Design review of the part built by this model. Coordinates are the model's own, in mm. A direction names the side the tool comes from. Give positions to 0.01 mm unless a question says otherwise; leave off trailing zeros. Order: outer loops, then holes, each group sorted by start corner. A loop starts at its lowest first (then second) coordinate and runs counter-clockwise, first axis right, second up. Notation, with made-up numbers: (26.25, 6.25) -> (34.25, 6.25) arc R16 ccw to (34.25, 35.25) -> close; hole circle Ø4 at (13, 5). An arc over 180 degrees is marked (long way). One line per item, written item: value. Start each with the question number.
1) Consider section B-B (z = 87.5). State the section outline as (x, y) points, plus the area to 3 significant figures.
2) The part is to be moulded in two halves that separate along X. For faces 4 (the face through (16.421, -2.535, 26.862)), 5 (the face through (11.68, -1.36, 7)), 6 (the face through (5.625, -3, 44)), say which applies: released by +X, released by -X, zero draft, split by the parting line, or undercut.
3) Tool access review of faces 1 (the face through (12.47, -2.535, 73.859)), 2 (the face through (12.47, -2.465, 86.792)), 3 (the face through (5.625, -2, 80)): name each direction out of +Z, -Z, +X, -X, +Y, -Y from which nothing blocks a thin tool from reaching the whole face with its end or side.
4) Wall thickness on line 1 along Z through (x, y) = (2.5, -3.2); line 2 along Z through (x, y) = (2, -4.25); line 3 along Z through (x, y) = (13, -1.2): over which ranges is each line inside the solid? List them lowest first. Write a range as from..to.
5) Consider section C-C (x = 15). State how many separate pieces and enclosed holes the cut face has, plus the area to 3 significant figures.
6) For pin 1 (2.5 mm diameter, centred on y = -2.5, z = 43.5, fed in from +X); pin 2 (8 mm diameter, centred on x = 14.5, z = 76.5, fed in from +Y); pin 3 (1.2 mm diameter, centred on x = 2.63, z = 11.83, fed in from +Y); pin 4 (4 mm diameter, centred on x = 12.38, z = 8.33, fed in from -Y), all flat-tipped, find the tip position at first contact; note any pin that passes through.
7) Consider section D-D (z = 65). State the section outline as (x, y) points, plus the area to 3 significant figures.
8) Consider section A-A (x = 7.25). State the section outline as (y, z) points.
from build123d import *

# Parameters (mm, degrees)
F1_DEPTH        = 5
F4_DEPTH        = 13.5
F6_DEPTH        = 7.5
F8_DEPTH        = 6.5
F10_D           = 3
F10_CSINK_D     = 7.5
F10_CSINK_ANGLE = 90
F12_D           = 2
F12_CSINK_D     = 5
F12_CSINK_ANGLE = 90


with BuildPart() as f1:
    # F0 (on Front) → F1 (new body)
    with BuildSketch(Plane.XZ):
        Polygon((19.12546, 114.327021), (-0.37454, 114.327021), (-0.37454, -0.672979), (19.62546, -0.672979), (19.62546, 29.327021), (13.12546, 29.327021), (13.12546, 39.827021), (5.62546, 39.827021), (5.62546, 48.327021), (19.12546, 48.327021), (19.12546, 75.827021), (5.62546, 75.827021), (5.62546, 84.327021), (19.12546, 84.327021), align=None)
    extrude(amount=F1_DEPTH)

    # F2 (on face) + F3 (on face) → F4 (cut)
    with BuildSketch(Plane.YZ.offset(19.12546)):
        Polygon((-5, 84.327021), (0, 84.327021), (-5, 89.327021), align=None)
    with BuildSketch(Plane.YZ.offset(19.12546)):
        Polygon((0, 75.827021), (-5, 75.827021), (0, 71.834676), align=None)
        Polygon((0, 53.327021), (-5, 48.327021), (0, 48.327021), align=None)
    extrude(amount=-F4_DEPTH, mode=Mode.SUBTRACT)

    # F5 (on face) → F6 (cut)
    with BuildSketch(Plane.YZ.offset(13.12546)):
        Polygon((-5, 34.827021), (0, 39.827021), (-5, 39.827021), align=None)
    extrude(amount=-F6_DEPTH, mode=Mode.SUBTRACT)

    # F7 (on face) → F8 (cut)
    with BuildSketch(Plane.YZ.offset(19.62546)):
        Polygon((0, 24.327021), (0, 29.327021), (-5, 29.327021), align=None)
    extrude(amount=-F8_DEPTH, mode=Mode.SUBTRACT)

    # F10 (through all)
    with Locations(Plane.XZ.offset(5)):
        with Locations((12.37546, 105.327021), (12.37546, 8.327021)):
            CounterSinkHole(F10_D / 2, F10_CSINK_D / 2, counter_sink_angle=F10_CSINK_ANGLE)

    # F12 (through all)
    with Locations(Plane(origin=(0, 0, 0), x_dir=(-1, 0, 0), z_dir=(0, 1, 0))):
        with Locations((-2.62546, 11.827021), (-2.62546, 99.327021)):
            CounterSinkHole(F12_D / 2, F12_CSINK_D / 2, counter_sink_angle=F12_CSINK_ANGLE)


solid = f1.part
Checked values:
1. outline: (-0.37, -5) -> (5.63, -5) -> (5.63, -3.17) -> (19.13, -3.17) -> (19.13, 0) -> (-0.37, 0) -> close
1. area: 72.8 mm^2
2. face 4: zero draft
2. face 5: undercut
2. face 6: released by +X
3. face 1: +X, +Y
3. face 2: +X, -Y
3. face 3: +X
4. line 1: z = -0.67..10.83, 12.82..98.33, 100.32..114.33
4. line 2: z = -0.67..11.05, 12.61..98.55, 100.11..114.33
4. line 3: z = -0.67..6.96, 9.69..38.63, 52.13..72.79, 85.53..103.96, 106.69..114.33
5. separate pieces: 3
5. enclosed holes: 0
5. area: 382 mm^2
6. pin 1: stops at x = 5.63
6. pin 2: stops at y = -0.83
6. pin 3: passes through
6. pin 4: stops at y = -3.26
7. outline: (-0.37, -5) -> (19.13, -5) -> (19.13, 0) -> (-0.37, 0) -> close
7. area: 97.5 mm^2
8. outline: (-5, -0.67) -> (0, -0.67) -> (0, 39.83) -> (-5, 34.83) -> close; (-5, 48.33) -> (0, 53.33) -> (0, 71.83) -> (-5, 75.83) -> close; (-5, 89.33) -> (0, 84.33) -> (0, 114.33) -> (-5, 114.33) -> close
